from build123d import *

# Parameters (mm, degrees)
F0_W     = 50.8
F0_H     = 50.8
F1_DEPTH = 152.4
F2_W     = 44.45
F2_H     = 44.45
F3_DEPTH = 876.3
F4_R     = 9.525
F6_D     = 12.7
F6_DEPTH = 127


with BuildPart() as f1:
    # F0 (on Right) → F1 (new body)
    with BuildSketch(Plane.YZ):
        with Locations((25.4, 25.4)):
            Rectangle(F0_W, F0_H)
    extrude(amount=-F1_DEPTH)

    # F2 (on face) → F3 (cut)
    with BuildSketch(Plane.YZ):
        with Locations((25.4, 25.4)):
            Rectangle(F2_W, F2_H)
    extrude(amount=-F3_DEPTH, mode=Mode.SUBTRACT)

    # F4
    f4_edges = [f1.edges().sort_by_distance(p)[0] for p in [
        (-76.2, 3.175, 3.175),
        (-76.2, 47.625, 3.175),
        (-76.2, 47.625, 47.625),
        (-76.2, 3.175, 47.625),
        (-76.2, 50.8, 0),
        (-76.2, 50.8, 50.8),
        (-76.2, 0, 50.8),
        (-76.2, 0, 0),
    ]]
    fillet(f4_edges, radius=F4_R)

    # F6
    with Locations(Plane.XZ):
        with Locations((-88.9, 25.4)):
            Hole(F6_D / 2, depth=F6_DEPTH)


solid = f1.part
Can you work these out from the model? Positions are in its coordinate system, mm. A direction names the side the tool comes from. Give positions to 0.01 mm unless a question says otherwise; leave off trailing zeros. Order: outer loops, then holes, each group sorted by start corner. A loop starts at its lowest first (then second) coordinate and runs counter-clockwise, first axis right, second up. Notation, with made-up numbers: (-16, 87) - (-8, 87) arc R9 cw to (-8, 91) - close; hole circle Ø5 at (15, 67.5). An arc over 180 degrees is marked (long way). Write each question's results on one line, items separated by ' | '.
1) Suppose I cut it at A-A, the plane z = 25.4. Write out the boundary of the cut face in (x, y) (3 decimals).
Final values:
outline: (-152.4, 0) - (-95.25, 0) - (-95.25, 3.175) - (-152.4, 3.175) - close; (-152.4, 47.625) - (-95.25, 47.625) - (-95.25, 50.8) - (-152.4, 50.8) - close; (-82.55, 0) - (0, 0) - (0, 3.175) - (-82.55, 3.175) - close; (-82.55, 47.625) - (0, 47.625) - (0, 50.8) - (-82.55, 50.8) - close
2) Please list where these lines run through material, in increasing order: line 1 along Y through (x, z) = (-64.5, 36) (3 decimals); line 2 along Z through (x, y) = (-69, 12.5); line 3 along X through (y, z) = (48, 25). Write a range as [from, to].
Final values:
line 1: y = [0, 3.175], [47.625, 50.8] | line 2: z = [0, 3.18], [47.62, 50.8] | line 3: x = [-152.4, -95.24], [-82.56, 0]
3) Suppose I cut it at B-B, the plane y = 31. Write out the boundary of the cut face in (x, z) (3 decimals), then the cut area to 3 significant figures.
Final values:
outline: (-152.4, 0) - (0, 0) - (0, 3.175) - (-152.4, 3.175) - close; (-152.4, 47.625) - (0, 47.625) - (0, 50.8) - (-152.4, 50.8) - close | area: 968 mm^2
4) I'm going to push a flat-ended pin straight in: pin 1 Ø1 at (x, y) = (-71, 5.5) entering from +Z. Where does the tip first touch, or does it pass through?
Final values:
pin 1: stops at z = 50.12
5) Suppose I cut it at C-C, the plane x = -88.9. Write out the boundary of the cut face in (y, z) (3 decimals).
Final values:
outline: (0, 9.525) arc R9.525 ccw to (9.525, 0) - (41.275, 0) arc R9.525 ccw to (50.8, 9.525) - (50.8, 19.05) - (47.625, 19.05) - (47.625, 12.7) arc R9.525 cw to (38.1, 3.175) - (12.7, 3.175) arc R9.525 cw to (3.175, 12.7) - (3.175, 19.05) - (0, 19.05) - close; (0, 31.75) - (3.175, 31.75) - (3.175, 38.1) arc R9.525 cw to (12.7, 47.625) - (38.1, 47.625) arc R9.525 cw to (47.625, 38.1) - (47.625, 31.75) - (50.8, 31.75) - (50.8, 41.275) arc R9.525 ccw to (41.275, 50.8) - (9.525, 50.8) arc R9.525 ccw to (0, 41.275) - close
6) If we mould it in two halves opening along Y, with no side actions, what happens to faces 1 (the face through (-82.556, 49.235, 25.679)), 2 (the face through (-77.27, 44.91, 44.76)), 3 (the face through (-77.27, 47.94, 2.72))? For each: pulls with the +Y half, pulls with the -Y half, needs draft (parallel to the pull), parting line crosses it, or undercut.
Final values:
face 1: needs draft | face 2: undercut | face 3: pulls with the +Y half
7) On a 3-axis mill with a long thin cutter (end or side, diameter ignored), from which of +Z, -Z, +X, -X, +Y, -Y can I reach the whole of each face in a straight line? I mean faces 4 (the face through (-77.27, 2.72, 2.86)), 5 (the face through (-75, 47.625, 25)). Say none if no direction works.
Final values:
face 4: -Z, +X, -X, -Y | face 5: +X, -X
8) Suppose I cut it at D-D, the plane x = -125.5. Write out the boundary of the cut face in (y, z) (3 decimals).
Final values:
outline: (0, 9.525) arc R9.525 ccw to (9.525, 0) - (41.275, 0) arc R9.525 ccw to (50.8, 9.525) - (50.8, 41.275) arc R9.525 ccw to (41.275, 50.8) - (9.525, 50.8) arc R9.525 ccw to (0, 41.275) - close; hole (3.175, 12.7) arc R9.525 ccw to (12.7, 3.175) - (38.1, 3.175) arc R9.525 ccw to (47.625, 12.7) - (47.625, 38.1) arc R9.525 ccw to (38.1, 47.625) - (12.7, 47.625) arc R9.525 ccw to (3.175, 38.1) - close
